Geometry check sheet. Reference: the model listing, model coordinates, mm. A direction names the side the tool comes from. Coordinates: 2 decimals unless noted, no trailing zeros. Order: outer loops, then holes, each group sorted by start corner. A loop starts at its lowest first (then second) coordinate and runs counter-clockwise, first axis right, second up. Notation, with made-up numbers: M 74,88 L 125,88 A9 cw 125,94 Z; hole C -21.75,26.5 d8. An arc over 180 degrees is marked long. Use CSV: the item, a comma, the result in double quotes. Start each with the question number.
```python
from build123d import *

# Parameters (mm, degrees)
SKETCH1_R           = 1.65
BOSS_EXTRUDE1_DEPTH = 7
CHAMFER1_SIZE       = 40
CHAMFER1_SIZE2      = 2.797072478
SKETCH2_R           = 1.3
CUT_EXTRUDE1_DEPTH  = 144.073407732
SKETCH3_R           = 1.3
CUT_EXTRUDE2_DEPTH  = 144.073407732
CUT_EXTRUDE3_DEPTH  = 3
CUT_EXTRUDE4_DEPTH  = 2
SKETCH6_W           = 4
SKETCH6_H           = 33.4
CUT_EXTRUDE5_DEPTH  = 144.073407732


with BuildPart() as part:
    # Sketch1 → Boss-Extrude1 (new body)
    with BuildSketch(Plane(origin=(0, 0, 0), x_dir=(1, 0, 0), z_dir=(0, 1, 0))):
        with BuildLine():
            Line((0, 0), (90, 0))
            Line((90, 0), (90, 61))
            Line((90, 61), (75, 61))
            ThreePointArc((75, 61), (69.343145751, 63.343145751), (67, 69))
            Line((67, 69), (67, 111))
            Line((67, 111), (23, 111))
            Line((23, 111), (23, 69))
            ThreePointArc((23, 69), (20.656854249, 63.343145751), (15, 61))
            Line((15, 61), (0, 61))
            Line((0, 61), (0, 0))
        make_face()
        with Locations(Location((3.725, 57.525, 0), (0, 0, 270))):
            Circle(SKETCH1_R, mode=Mode.SUBTRACT)
        with Locations(Location((86.275, 57.525, 0), (0, 0, 270))):
            Circle(SKETCH1_R, mode=Mode.SUBTRACT)
        with Locations(Location((86.275, 3.475, 0), (0, 0, 270))):
            Circle(SKETCH1_R, mode=Mode.SUBTRACT)
        with Locations(Location((3.725, 3.475, 0), (0, 0, 270))):
            Circle(SKETCH1_R, mode=Mode.SUBTRACT)
    extrude(amount=BOSS_EXTRUDE1_DEPTH)

    # Chamfer1
    chamfer1_edges = [part.edges().sort_by_distance(p)[0] for p in [
        (45, 0, -111),
    ]]
    chamfer1_side = [part.faces().sort_by_distance(p)[0] for p in [
        (45, 0, -46.507129493),
    ]]
    chamfer(chamfer1_edges, length=CHAMFER1_SIZE, length2=CHAMFER1_SIZE2, reference=chamfer1_side[0])

    # Sketch2 → Cut-Extrude1 (cut, through all)
    with BuildSketch(Plane(origin=(0, 7, 0), x_dir=(1, 0, 0), z_dir=(0, 1, 0))):
        with Locations(Location((8, 52.5, 0), (0, 0, 270))):
            Circle(SKETCH2_R)
        with Locations(Location((8, 8.5, 0), (0, 0, 270))):
            Circle(SKETCH2_R)
        with Locations(Location((82, 52.5, 0), (0, 0, 270))):
            Circle(SKETCH2_R)
        with Locations(Location((82, 8.5, 0), (0, 0, 270))):
            Circle(SKETCH2_R)
    extrude(amount=-CUT_EXTRUDE1_DEPTH, mode=Mode.SUBTRACT)

    # Sketch3 → Cut-Extrude2 (cut, through all)
    with BuildSketch(Plane(origin=(0, 7, 0), x_dir=(1, 0, 0), z_dir=(0, 1, 0))):
        with Locations(Location((26, 106, 0), (0, 0, 270))):
            Circle(SKETCH3_R)
        with Locations(Location((64, 106, 0), (0, 0, 270))):
            Circle(SKETCH3_R)
        with Locations(Location((26, 66, 0), (0, 0, 270))):
            Circle(SKETCH3_R)
        with Locations(Location((64, 66, 0), (0, 0, 270))):
            Circle(SKETCH3_R)
    extrude(amount=-CUT_EXTRUDE2_DEPTH, mode=Mode.SUBTRACT)

    # Sketch4 → Cut-Extrude3 (cut)
    with BuildSketch(Plane(origin=(0, 7, 0), x_dir=(1, 0, 0), z_dir=(0, 1, 0))):
        with BuildLine():
            Line((12, 52.5), (78, 52.5))
            ThreePointArc((78, 52.5), (79.171572875, 49.671572875), (82, 48.5))
            Line((82, 48.5), (82, 12.5))
            ThreePointArc((82, 12.5), (79.171572875, 11.328427125), (78, 8.5))
            Line((78, 8.5), (12, 8.5))
            ThreePointArc((12, 8.5), (10.828427125, 11.328427125), (8, 12.5))
            Line((8, 12.5), (8, 48.5))
            ThreePointArc((8, 48.5), (10.828427125, 49.671572875), (12, 52.5))
        make_face()
    extrude(amount=-CUT_EXTRUDE3_DEPTH, mode=Mode.SUBTRACT)

    # Sketch5 → Cut-Extrude4 (cut)
    with BuildSketch(Plane(origin=(0, 7, 0), x_dir=(1, 0, 0), z_dir=(0, 1, 0))):
        with BuildLine():
            Line((29.3, 106), (60.7, 106))
            ThreePointArc((60.7, 106), (61.666547622, 103.666547622), (64, 102.7))
            Line((64, 102.7), (64, 69.3))
            ThreePointArc((64, 69.3), (61.666547622, 68.333452378), (60.7, 66))
            Line((60.7, 66), (29.3, 66))
            ThreePointArc((29.3, 66), (28.333452378, 68.333452378), (26, 69.3))
            Line((26, 69.3), (26, 102.7))
            ThreePointArc((26, 102.7), (28.333452378, 103.666547622), (29.3, 106))
        make_face()
    extrude(amount=-CUT_EXTRUDE4_DEPTH, mode=Mode.SUBTRACT)

    # Sketch6 → Cut-Extrude5 (cut, through all)
    with BuildSketch(Plane(origin=(0, 7, 0), x_dir=(1, 0, 0), z_dir=(0, 1, 0))):
        with Locations((25, 86)):
            Rectangle(SKETCH6_W, SKETCH6_H)
        with Locations((65, 86)):
            Rectangle(SKETCH6_W, SKETCH6_H)
    extrude(amount=-CUT_EXTRUDE5_DEPTH, mode=Mode.SUBTRACT)


solid = part.part
```
1) Section check A-A on z = -14. Record the boundary of the cut face in (x, y).
2) Section check C-C on x = 73. Record the boundary of the cut face in (y, z), then the cut area to 3 significant figures.
3) Material ranges on line 1 along X through (y, z) = (2.25, -8.5); line 2 along Z through (x, y) = (48, 5.5); line 3 along Z through (x, y) = (64, 5.5), recorded low to high.
4) Section check D-D on z = -90. Record the boundary of the cut face in (x, y).
5) Section check B-B on x = 33. Record the boundary of the cut face in (y, z).
6) Draft check along Z on faces 1 (the face through (63.5, 4.7, -104.8)), 2 (the face through (8, 6, -30)), 3 (the face through (90, 3, -30)), 4 (the face through (44, 3, 0)). Enter one of: +Z half, -Z half, draft (parallel to the pull), parting line (faces both ways), or undercut.
7) Gauge pin test, flat ends, axial feed: P1, Ø3.5, axis at x = 86, y = 3, coming from the -Z side; P2, Ø1.6, axis at x = 8, z = -8.5, coming from the +Y side; P3, Ø8, axis at x = 33.5, z = -97, coming from the -Y side; P4, Ø3, axis at x = 64, z = -106, coming from the -Y side. Record the tip position at first contact, or that the pin passes through.
8) Set-up check for faces 5 (the face through (65, 4, -69.3)), 6 (the face through (61.641, 6.014, -103.692)), 7 (the face through (25.5, 3.5, -64.8)): record each of +Z, -Z, +X, -X, +Y, -Y from which the full face is reachable in a straight line by a thin tool's end or side.
Results are:
1,outline,"M 0,0 L 90,0 L 90,7 L 82,7 L 82,4 L 8,4 L 8,7 L 0,7 Z"
2,outline,"M 0,-61.25 L 7,-61.25 L 7,-52.5 L 4,-52.5 L 4,-8.5 L 7,-8.5 L 7,0 L 0,0 Z"
2,area,"297 mm²"
3,line 1,"x = 0 to 6.7, 9.3 to 80.7, 83.3 to 90"
3,line 2,"z = -111 to -106, -66 to -52.5, -8.5 to 0"
3,line 3,"z = -111 to -107.3, -104.7 to -102.7, -69.3 to -67.3, -64.7 to -52.5, -8.5 to 0"
4,outline,"M 27,1.33 L 63,1.33 L 63,5 L 27,5 Z"
5,outline,"M 0,-71 L 2.8,-111 L 7,-111 L 7,-106 L 5,-106 L 5,-66 L 7,-66 L 7,-52.5 L 4,-52.5 L 4,-8.5 L 7,-8.5 L 7,0 L 0,0 Z"
6,face 1,"undercut"
6,face 2,"undercut"
6,face 3,"draft"
6,face 4,"+Z half"
7,P1,"stops at z = -61"
7,P2,"passes through"
7,P3,"stops at y = 1.54"
7,P4,"stops at y = 2.34"
8,face 5,"+X, +Y, -Y"
8,face 6,"+Y"
8,face 7,"+Y, -Y"
